```python
from build123d import *

# Parameters (mm, degrees)
SKETCH1_R               = 30
BOSS_EXTRUDE1_DEPTH     = 25
CUT_EXTRUDE1_DEPTH      = 1
CUT_EXTRUDE1_DEPTH_BACK = 43
SKETCH2_R               = 5
SKETCH3_W               = 1.5
SKETCH3_H               = 1.5
SKETCH5_R               = 10
BOSS_EXTRUDE2_DEPTH     = 3
SKETCH6_R               = 5
CUT_EXTRUDE3_DEPTH      = 3
CUT_EXTRUDE4_START      = -38
CUT_EXTRUDE4_DEPTH      = 38


with BuildPart() as part:
    # Sketch1 → Boss-Extrude1 (new body)
    with BuildSketch(Plane.XY):
        Circle(SKETCH1_R)
    extrude(amount=BOSS_EXTRUDE1_DEPTH)

    # Sketch2 → Cut-Extrude1 (cut, two sides: drawn at the far end of the back side and taken through both)
    with BuildSketch(Plane.XY.offset(25).offset(-CUT_EXTRUDE1_DEPTH_BACK)):
        Circle(SKETCH2_R)
    extrude(amount=CUT_EXTRUDE1_DEPTH + CUT_EXTRUDE1_DEPTH_BACK, mode=Mode.SUBTRACT)

    # Sketch3 → Cut-Revolve2 (revolve, cut)
    with BuildSketch(Plane(origin=(0, 0, 0), x_dir=(0, 0, -1), z_dir=(1, 0, 0)), mode=Mode.PRIVATE) as cut_revolve2_sk:
        with Locations((-12.5, 30)):
            Rectangle(SKETCH3_W, SKETCH3_H)
        with Locations((-8.5, 30)):
            Rectangle(SKETCH3_W, SKETCH3_H)
        with Locations((-4.5, 30)):
            Rectangle(SKETCH3_W, SKETCH3_H)
        with Locations((-16.5, 30)):
            Rectangle(SKETCH3_W, SKETCH3_H)
        with Locations((-20.5, 30)):
            Rectangle(SKETCH3_W, SKETCH3_H)
    revolve(cut_revolve2_sk.sketch.rotate(Axis((0, 0, 25), (0, 0, -1)), 90), axis=Axis((0, 0, 25), (0, 0, -1)), mode=Mode.SUBTRACT)

    # Sketch5 → Boss-Extrude2 (add)
    with BuildSketch(Plane.XY.offset(25)):
        Circle(SKETCH5_R)
    extrude(amount=BOSS_EXTRUDE2_DEPTH)

    # Sketch6 → Cut-Extrude3 (cut)
    with BuildSketch(Plane.XY.offset(28)):
        Circle(SKETCH6_R)
    extrude(amount=-CUT_EXTRUDE3_DEPTH, mode=Mode.SUBTRACT)

    # Sketch7 → Cut-Extrude4 (cut)
    with BuildSketch(Plane(origin=(0, 0, 0), x_dir=(-1, 0, 0), z_dir=(0, 0, -1)).offset(CUT_EXTRUDE4_START)):
        with BuildLine():
            Line((-1.5, 6.419696007), (1.5, 6.419696007))
            Line((1.5, 6.419696007), (1.5, 4.769696007))
            ThreePointArc((1.5, 4.769696007), (0, 5), (-1.5, 4.769696007))
            Line((-1.5, 4.769696007), (-1.5, 6.419696007))
        make_face()
    extrude(amount=CUT_EXTRUDE4_DEPTH, mode=Mode.SUBTRACT)


solid = part.part
```
The model under review builds one solid part; all positions refer to its coordinate system, in mm. A direction names the side the tool comes from. Round coordinates to 2 decimals unless told otherwise and drop trailing zeros. Use CSV: the item, a comma, the result in double quotes. Start each with the question number.
(1) For line 1 along Z through (x, y) = (25, 15.5); line 2 along Y through (x, z) = (0, 22); line 3 along X through (y, z) = (0, 15.25), list the stretches that pass through material, from the lowest coordinate up.
(2) The part is to be moulded in two halves that separate along X. For faces 1 (the face through (-29.97, 1.32, 23.1)), 2 (the face through (0, 6.42, 14)), 3 (the face through (1.5, 6, 14)), 4 (the face through (6, 0, 0)), say which applies: +X half, -X half, draft (parallel to the pull), parting line (faces both ways), or undercut.
(3) Clearance check with flat-ended pins moving along their axes: P1, Ø8, axis at y = 22, z = 19, coming from the +X side; P2, Ø4, axis at x = 8.5, y = -20, coming from the +Z side; P3, Ø0.5, axis at y = 5.5, z = 19.5, coming from the -X side; P4, Ø4, axis at x = -13, y = 9.5, coming from the -Z side. State where each tip first meets the part, or that it passes through.
(4) Tool access review of faces 5 (the face through (13, 0, 25)), 6 (the face through (-1.5, 6, 14)), 7 (the face through (-29, 7, 19.75)): name each direction out of +Z, -Z, +X, -X, +Y, -Y from which nothing blocks a thin tool from reaching the whole face with its end or side.
Findings:
1,line 1,"0 to 3.75, 5.25 to 7.75, 9.25 to 11.75, 13.25 to 15.75, 17.25 to 19.75, 21.25 to 25"
1,line 2,"-30 to -5, 6.42 to 30"
1,line 3,"-30 to -5, 5 to 30"
2,face 1,"parting line"
2,face 2,"undercut"
2,face 3,"undercut"
2,face 4,"draft"
3,P1,"x = 24"
3,P2,"z = 25"
3,P3,"x = -29.54"
3,P4,"z = 0"
4,face 5,"+Z"
4,face 6,"+Z, -Z"
4,face 7,"none"
